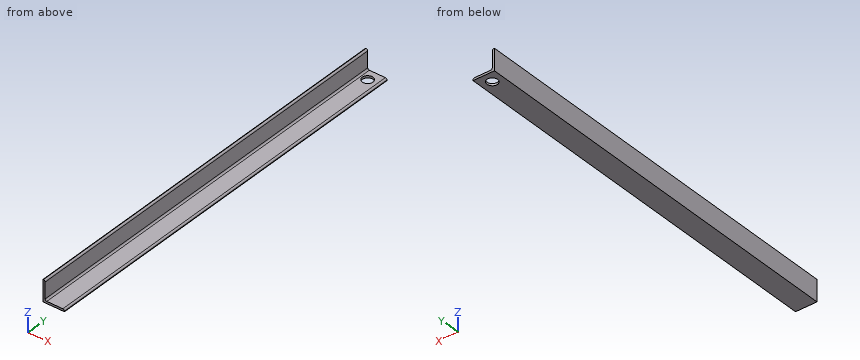
from build123d import *

# Parameters (mm, degrees)
BOSS_EXTRUDE1_DEPTH = 750
SKETCH2_R           = 10
CUT_EXTRUDE1_DEPTH  = 754.891393199


with BuildPart() as part:
    # Sketch1 → Boss-Extrude1 (new body)
    with BuildSketch(Plane(origin=(0, 0, 0), x_dir=(1, 0, 0), z_dir=(0, 1, 0))):
        with BuildLine():
            Line((-27.499872145, 29.213153277), (-67.499872145, 29.213153277))
            Line((-67.499872145, 29.213153277), (-67.499872145, -10.786846723))
            Line((-67.499872145, -10.786846723), (-66.499872145, -10.786846723))
            ThreePointArc((-66.499872145, -10.786846723), (-64.378551801, -9.908167067), (-63.499872145, -7.786846723))
            Line((-63.499872145, -7.786846723), (-63.499872145, 22.213153277))
            ThreePointArc((-63.499872145, 22.213153277), (-62.621192489, 24.334473621), (-60.499872145, 25.213153277))
            Line((-60.499872145, 25.213153277), (-30.499872145, 25.213153277))
            ThreePointArc((-30.499872145, 25.213153277), (-28.378551801, 26.091832933), (-27.499872145, 28.213153277))
            Line((-27.499872145, 28.213153277), (-27.499872145, 29.213153277))
        make_face()
    extrude(amount=BOSS_EXTRUDE1_DEPTH)

    # Sketch2 → Cut-Extrude1 (cut, through all)
    with BuildSketch(Plane.XY.offset(-25.213153277)):
        with Locations((-47.499872145, 730)):
            Circle(SKETCH2_R)
    extrude(amount=-CUT_EXTRUDE1_DEPTH, mode=Mode.SUBTRACT)


solid = part.part
Geometry check sheet. Reference: the model listing, model coordinates, mm. Give positions to 0.01 mm unless a question says otherwise; leave off trailing zeros. Loops run counter-clockwise (first coordinate to the right, second up) from the corner with the lowest first, then second, coordinate; pieces in that order, holes last. Notation, with made-up numbers: (-37, 83) -> (-5, 83) arc R24 ccw to (-5, 117) -> close; hole circle Ø5 at (-6, -19.5). An arc over 180 degrees is marked (long way). Answer in a Markdown table with one row per item. Add a question column.
1) Cross-section at A-A on y = 730. Record the boundary of the cut face in (x, z).
2) Material ranges on probe 1 along Z at (x, y) = (-45, 316); probe 2 along X at (y, z) = (730, -27.7); probe 3 along X at (y, z) = (328, -6), recorded low to high. Write a range as from..to.
3) Cross-section at B-B on y = 103. Record the boundary of the cut face in (x, z), and give its area (3 significant figures).
4) Cross-section at C-C on z = -11. Record the boundary of the cut face in (x, y).
5) Gauge pin test, flat ends, axial feed: P1, Ø3, axis at x = -36, y = 293, coming from the +Z side; P2, Ø24, axis at y = 208, z = -9.5, coming from the +X side. Record the tip position at first contact, or that the pin passes through.
Outcome:
| question | item | result |
|---|---|---|
| 1 | outline | (-67.5, -29.21) -> (-57.5, -29.21) -> (-57.5, -25.21) -> (-60.5, -25.21) arc R3 cw to (-63.5, -22.21) -> (-63.5, 7.79) arc R3 ccw to (-66.5, 10.79) -> (-67.5, 10.79) -> close; (-37.5, -29.21) -> (-27.5, -29.21) -> (-27.5, -28.21) arc R3 ccw to (-30.5, -25.21) -> (-37.5, -25.21) -> close |
| 2 | probe 1 | z = -29.21..-25.21 |
| 2 | probe 2 | x = -67.5..-57.5, -37.5..-27.54 |
| 2 | probe 3 | x = -67.5..-63.5 |
| 3 | outline | (-67.5, -29.21) -> (-27.5, -29.21) -> (-27.5, -28.21) arc R3 ccw to (-30.5, -25.21) -> (-60.5, -25.21) arc R3 cw to (-63.5, -22.21) -> (-63.5, 7.79) arc R3 ccw to (-66.5, 10.79) -> (-67.5, 10.79) -> close |
| 3 | area | 302 mm^2 |
| 4 | outline | (-67.5, 0) -> (-63.5, 0) -> (-63.5, 750) -> (-67.5, 750) -> close |
| 5 | P1 | stops at z = -25.21 |
| 5 | P2 | stops at x = -63.5 |
